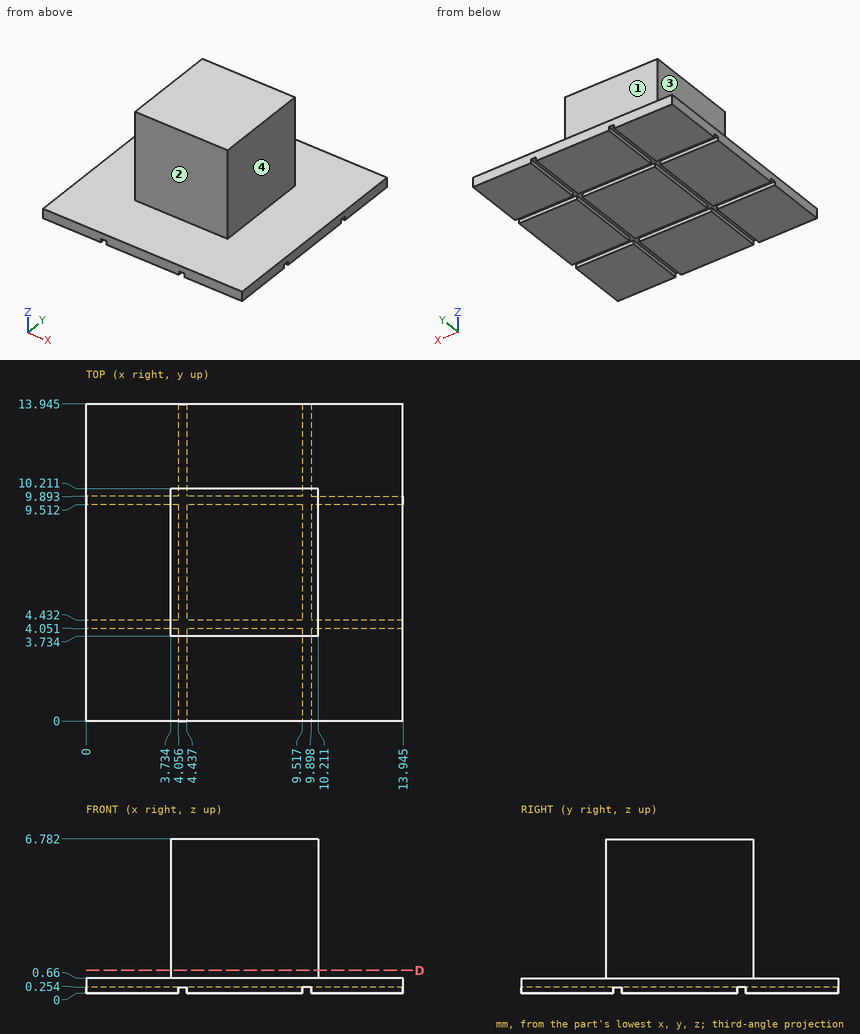
The figure shows three views and two pictorial views of one solid part (mm, origin at its lowest corner). Answer the questions. A direction names the side the tool comes from. Coordinates: 2 decimals unless noted, no trailing zeros. Loops run counter-clockwise (first coordinate to the right, second up) from the corner with the lowest first, then second, coordinate; pieces in that order, holes last. Notation, with made-up numbers: (57, -39) - (80, -39) arc R12 cw to (80, -16) - close; hole circle Ø6 at (-13, 79). An arc over 180 degrees is marked (long way). Use a Markdown table: item, result. Add a question column.
1) Given pin 1 (2 mm diameter, centred on y = 12, z = 5.5, fed in from -X); pin 2 (1 mm diameter, centred on y = 7, z = 5, fed in from +X); pin 3 (1.8 mm diameter, centred on x = 7.5, z = 3.5, fed in from +Y), each flat-ended and moving along its own axis, determine where each tip first touches the part or whether it passes through.
2) For the marked faces 1, 2, 3 and 4, determine the directions among +Z, -Z, +X, -X, +Y, -Y from which every point of the face is accessible in a straight line to the end or side of a thin tool.
3) Find the intervals of material crossed by line 1 (Z direction, x = 6.75, y = 1.75); line 2 (X direction, y = 6.5, z = 5.25), in increasing order.
4) The part is cut by section D-D, the plane z = 1. Give the vertices of the cut face in (x, y).
Here are the results:
| question | item | result |
|---|---|---|
| 1 | pin 1 | passes through |
| 1 | pin 2 | stops at x = 10.21 |
| 1 | pin 3 | stops at y = 10.21 |
| 2 | face 1 | +Z, +X, -X, +Y |
| 2 | face 2 | +Z, +X, -X, -Y |
| 2 | face 3 | +Z, -X, +Y, -Y |
| 2 | face 4 | +Z, +X, +Y, -Y |
| 3 | line 1 | z = 0 to 0.66 |
| 3 | line 2 | x = 3.73 to 10.21 |
| 4 | outline | (3.73, 3.73) - (10.21, 3.73) - (10.21, 10.21) - (3.73, 10.21) - close |
